from build123d import *

# Parameters (mm, degrees)
CROQUIS1_W                          = 15
CROQUIS1_H                          = 8
SALIENTE_EXTRUIR1_DEPTH             = 6.6
SALIENTE_EXTRUIR2_REACH             = 12.762
SALIENTE_EXTRUIR2_DIRECTION_2_REACH = 12.762
CROQUIS3_R                          = 1.75
CORTAR_EXTRUIR1_DEPTH               = 3
CORTAR_EXTRUIR2_DEPTH               = 0.25
MATRIZL1_COUNT                      = 3
MATRIZL1_PITCH                      = 5
CROQUIS5_R                          = 0.25
SALIENTE_EXTRUIR3_DEPTH             = 4
MATRIZL2_COUNT                      = 3
MATRIZL2_PITCH                      = 4.9
CROQUIS6_W                          = 4.3
CROQUIS6_H                          = 5.3
CROQUIS6_R                          = 1
CORTAR_EXTRUIR3_DEPTH               = 1.5
CROQUIS6_2_R                        = 1
CORTAR_EXTRUIR4_DEPTH               = 2
MATRIZL3_COUNT                      = 3
MATRIZL3_PITCH                      = 4.9


with BuildPart() as part:
    # Croquis1 → Saliente-Extruir1 (new body)
    with BuildSketch(Plane(origin=(0, 0, 0), x_dir=(1, 0, 0), z_dir=(0, 1, 0))):
        Rectangle(CROQUIS1_W, CROQUIS1_H)
    extrude(amount=SALIENTE_EXTRUIR1_DEPTH)

    # Saliente-Extruir2: up to this face of the body (flat: up to its plane)
    saliente_extruir2_end = Plane(part.part.faces().sort_by_distance((7.5, 3.3, 0))[0])
    # Croquis2 → Saliente-Extruir2 (add, up to the picked face)
    with BuildSketch(Plane(origin=(0, 0, 0), x_dir=(0, 0, -1), z_dir=(1, 0, 0)), mode=Mode.PRIVATE) as saliente_extruir2_sk1:
        Polygon((-4, 6.6), (4, 6.6), (2.3, 9.8), (-3.2, 9.8), align=None)
    saliente_extruir2_tool1 = split(extrude(saliente_extruir2_sk1.sketch, amount=SALIENTE_EXTRUIR2_REACH, mode=Mode.PRIVATE), bisect_by=saliente_extruir2_end, keep=Keep.BOTH, mode=Mode.PRIVATE)
    add(saliente_extruir2_tool1.solids().sort_by(Axis((0, 8.101235, 0.211111), (1, 0, 0)))[0])

    # Saliente-Extruir2 direction 2: up to this face of the body (flat: up to its plane)
    saliente_extruir2_direction_2_end = Plane(part.part.faces().sort_by_distance((-7.5, 3.3, 0))[0])
    # Croquis2 → Saliente-Extruir2 direction 2 (add, up to the picked face)
    with BuildSketch(Plane(origin=(0, 0, 0), x_dir=(0, 0, -1), z_dir=(1, 0, 0)), mode=Mode.PRIVATE) as saliente_extruir2_direction_2_sk1:
        Polygon((-4, 6.6), (4, 6.6), (2.3, 9.8), (-3.2, 9.8), align=None)
    saliente_extruir2_direction_2_tool1 = split(extrude(saliente_extruir2_direction_2_sk1.sketch, amount=-SALIENTE_EXTRUIR2_DIRECTION_2_REACH, mode=Mode.PRIVATE), bisect_by=saliente_extruir2_direction_2_end, keep=Keep.BOTH, mode=Mode.PRIVATE)
    add(saliente_extruir2_direction_2_tool1.solids().sort_by(Axis((0, 8.101235, 0.211111), (-1, 0, 0)))[0])

    # Croquis3 → Cortar-Extruir1 (cut)
    with BuildSketch(Plane(origin=(0, 9.8, 0), x_dir=(1, 0, 0), z_dir=(0, 1, 0))):
        with Locations(Location((-5.05, -0.45, 0), (0, 0, 270))):
            Circle(CROQUIS3_R)
    cortar_extruir1 = extrude(amount=-CORTAR_EXTRUIR1_DEPTH, mode=Mode.SUBTRACT)

    # Croquis4 → Cortar-Extruir2 (cut)
    with BuildSketch(Plane(origin=(0, 6.8, 0), x_dir=(1, 0, 0), z_dir=(0, 1, 0))):
        with BuildLine():
            ThreePointArc((-5.3, -2.182050808), (-5.05, -2.2), (-4.8, -2.182050808))
            Line((-4.8, -2.182050808), (-4.8, -0.7))
            Line((-4.8, -0.7), (-3.317949192, -0.7))
            ThreePointArc((-3.317949192, -0.7), (-3.304493066, -0.575321759), (-3.3, -0.45))
            ThreePointArc((-3.3, -0.45), (-3.304493066, -0.324678241), (-3.317949192, -0.2))
            Line((-3.317949192, -0.2), (-4.8, -0.2))
            Line((-4.8, -0.2), (-4.8, 1.282050808))
            ThreePointArc((-4.8, 1.282050808), (-5.05, 1.3), (-5.3, 1.282050808))
            Line((-5.3, 1.282050808), (-5.3, -0.2))
            Line((-5.3, -0.2), (-6.782050808, -0.2))
            ThreePointArc((-6.782050808, -0.2), (-6.8, -0.45), (-6.782050808, -0.7))
            Line((-6.782050808, -0.7), (-5.3, -0.7))
            Line((-5.3, -0.7), (-5.3, -2.182050808))
        make_face()
    cortar_extruir2 = extrude(amount=-CORTAR_EXTRUIR2_DEPTH, mode=Mode.SUBTRACT)

    # MatrizL1: Cortar-Extruir1, Cortar-Extruir2 ×3
    with Locations(*[(i * MATRIZL1_PITCH, 0, 0) for i in range(1, MATRIZL1_COUNT)]):
        add(cortar_extruir1, mode=Mode.SUBTRACT)
        add(cortar_extruir2, mode=Mode.SUBTRACT)

    # Croquis5 → Saliente-Extruir3 (add)
    with BuildSketch(Plane.XZ):
        with Locations(Location((-4.95, 0, 0), (0, 0, 90))):
            Circle(CROQUIS5_R)
    saliente_extruir3 = extrude(amount=SALIENTE_EXTRUIR3_DEPTH)

    # MatrizL2: Saliente-Extruir3 ×3
    with Locations(*[(i * MATRIZL2_PITCH, 0, 0) for i in range(1, MATRIZL2_COUNT)]):
        add(saliente_extruir3)

    # Croquis6 → Cortar-Extruir3 (cut)
    with BuildSketch(Plane.XY.offset(4)):
        with Locations((-4.85, 3.3)):
            Rectangle(CROQUIS6_W, CROQUIS6_H)
        with Locations((-4.85, 3.3)):
            Circle(CROQUIS6_R, mode=Mode.SUBTRACT)
    cortar_extruir3 = extrude(amount=-CORTAR_EXTRUIR3_DEPTH, mode=Mode.SUBTRACT)

    # Croquis6_2 → Cortar-Extruir4 (cut)
    with BuildSketch(Plane.XY.offset(4)):
        with Locations((-4.85, 3.3)):
            Circle(CROQUIS6_2_R)
    cortar_extruir4 = extrude(amount=-CORTAR_EXTRUIR4_DEPTH, mode=Mode.SUBTRACT)

    # MatrizL3: Cortar-Extruir3, Cortar-Extruir4 ×3
    with Locations(*[(i * MATRIZL3_PITCH, 0, 0) for i in range(1, MATRIZL3_COUNT)]):
        add(cortar_extruir3, mode=Mode.SUBTRACT)
        add(cortar_extruir4, mode=Mode.SUBTRACT)


solid = part.part
Build history of the part. All positions in model axes, mm. A direction names the side the tool comes from. Round coordinates to 2 decimals unless told otherwise and drop trailing zeros. Write each loop counter-clockwise with the first axis right and the second up, starting at its lowest first coordinate (ties: lowest second). Pieces come first, ordered by that corner, then holes. Notation, with made-up numbers: M 6,-18 L 41,-18 A28 ccw 41,20 Z; hole C 15,-13 d9. An arc over 180 degrees is marked long. Answer as a JSON object with one key per item and string values. Group by question number.
(1) Cut at B-B (y = -3). Give the cut face in (x, z).
(2) Cut at D-D (z = -0.5). Give the cut face in (x, y).
(3) Mould opens along X. For faces 1 (the flat face through (2.8, 3, 3)), 2 (the flat face through (2, 9.8, 0)), 3 (the flat face through (-7.5, 5, 0)) say: pulls with the +X half, pulls with the -X half, needs draft (parallel to the pull), parting line crosses it, or undercut.
(4) Drill centre lines: L1, parallel to X at y = 8.1, z = 0.45; L2, parallel to Y at x = -4, z = 3; L3, parallel to Y at x = 0.05, z = 2.15. Where is each one in solid material? Low to high.
(5) Cut at A-A (y = 3.3). Give the cut face in (x, z), and give its area (4 significant figures).
(6) Which spindle directions (+Z, -Z, +X, -X, +Y, -Y) get a long thin tool onto all of the face, cutting with end or side? Do faces 4 (the flat face through (-1, 6.8, 0)), 5 (the flat face through (-6, 3, 2.5)), 6 (the flat face through (0.11, 8.18, -3.16)). Say none if no direction does.
(7) Cut at C-C (x = -2.5). Give the cut face in (y, z).
(8) Flat gauge pins, fed straight in: pin 1 (3.5 mm diameter, centred on x = -4, y = 4, fed in from +Z); pin 2 (1 mm diameter, centred on x = -5, z = 0.5, fed in from +Y); pin 3 (1.5 mm diameter, centred on y = -2.5, z = -2.5, fed in from -X); pin 4 (1 mm diameter, centred on x = 4.5, y = 3, fed in from +Z). Where does each tip first touch, or does it go through?
Responses:
{
 "1": {"outline": "C -4.95,0 d0.5; C -0.05,0 d0.5; C 4.85,0 d0.5"},
 "2": {"outline": "M -7.5,0 L 7.5,0 L 7.5,9.8 L 6.42,9.8 L 6.42,6.8 L 5.2,6.8 L 5.2,6.55 L 4.7,6.55 L 4.7,6.8 L 3.48,6.8 L 3.48,9.8 L 1.42,9.8 L 1.42,6.8 L 0.2,6.8 L 0.2,6.55 L -0.3,6.55 L -0.3,6.8 L -1.52,6.8 L -1.52,9.8 L -3.58,9.8 L -3.58,6.8 L -4.8,6.8 L -4.8,6.55 L -5.3,6.55 L -5.3,6.8 L -6.52,6.8 L -6.52,9.8 L -7.5,9.8 Z"},
 "3": {"face 1": "undercut", "face 2": "needs draft", "face 3": "pulls with the -X half"},
 "4": {"L1": "x = -7.5 to -6.8, -3.3 to -1.8, 1.7 to 3.2, 6.7 to 7.5", "L2": "y = 0 to 0.65, 5.95 to 9.8", "L3": "y = 0 to 2.3, 4.3 to 6.55"},
 "5": {"outline": "M -7.5,-4 L 7.5,-4 L 7.5,4 L 7.1,4 L 7.1,2.5 L 5.95,2.5 L 5.95,2 L 3.95,2 L 3.95,2.5 L 2.8,2.5 L 2.8,4 L 2.2,4 L 2.2,2.5 L 1.05,2.5 L 1.05,2 L -0.95,2 L -0.95,2.5 L -2.1,2.5 L -2.1,4 L -2.7,4 L -2.7,2.5 L -3.85,2.5 L -3.85,2 L -5.85,2 L -5.85,2.5 L -7,2.5 L -7,4 L -7.5,4 Z", "area": "97.65 mm2"},
 "6": {"face 4": "+Y", "face 5": "+Z", "face 6": "-Z, +X, -X, +Y"},
 "7": {"outline": "M 0,-4 L 6.6,-4 L 9.8,-2.3 L 9.8,3.2 L 6.6,4 L 0,4 Z"},
 "8": {"pin 1": "stops at z = 4", "pin 2": "stops at y = 6.8", "pin 3": "passes through", "pin 4": "stops at z = 2.5"}
}
